Input: part model. Units: mm. Frame: model coordinates. A direction names the side the tool comes from. Give positions to 0.01 mm unless a question says otherwise; leave off trailing zeros. Loops run counter-clockwise (first coordinate to the right, second up) from the corner with the lowest first, then second, coordinate; pieces in that order, holes last. Notation, with made-up numbers: (35.5, 65.5) - (47.5, 65.5) arc R21 cw to (47.5, 91.5) - close; hole circle Ø3 at (39, 18.25). An arc over 180 degrees is marked (long way). Answer as a JSON object with one key per item and string values.
from build123d import *

# Parameters (mm, degrees)
SKETCH_2_R          = 2.5
CHAMFER_1_SIZE      = 10
CHAMFER_1_SIZE2     = 1.583844403
SKETCH_4_W          = 3.296860699
SKETCH_4_H          = 5.658889041
SKETCH_4_W_2        = 5.658889041
SKETCH_4_H_2        = 3.296860699
CUT_EXTRUDE_1_DEPTH = 40
DOME_1_FACE_RADIUS  = 0.916155597
DOME_1_HEIGHT       = 1


with BuildPart() as part:
    # 扫描1: sweep along a path in 草图1
    with BuildLine(Plane.XY) as sweep_1_path:
        Line((0, 0), (0, 34.641016151))
        ThreePointArc((0, 34.641016151), (0.681483474, 39.817397053), (2.679491924, 44.641016151))
        Line((2.679491924, 44.641016151), (17.5, 70.310889132))
    # 草图2 → 扫描1 (sweep)
    with BuildSketch(Plane(origin=(0, 0, 0), x_dir=(1, 0, 0), z_dir=(0, 1, 0))):
        Circle(SKETCH_2_R)
    sweep(path=sweep_1_path.line)

    # 草图3 → 旋转1 (revolve)
    with BuildSketch(Plane.XY, mode=Mode.PRIVATE) as revolve_1_sk:
        Polygon((0, 0), (2.5, 0), (4, -8), (4, -40), (0, -40), align=None)
    revolve(revolve_1_sk.sketch.rotate(Axis((0, 0, 0), (0, -1, 0)), 90), axis=Axis((0, 0, 0), (0, -1, 0)))

    # 倒角1
    chamfer_1_edges = [part.edges().sort_by_distance(p)[0] for p in [
        (15.334936491, 71.560889132, 0),
    ]]
    chamfer_1_side = [part.faces().sort_by_distance(p)[0] for p in [
        (7.924682453, 58.725952642, 0),
    ]]
    chamfer(chamfer_1_edges, length=CHAMFER_1_SIZE, length2=CHAMFER_1_SIZE2, reference=chamfer_1_side[0])

    # 草图4 → 切除-拉伸1 (cut)
    with BuildSketch(Plane.XZ.offset(40)):
        with Locations((5.148430349, -0.020531218)):
            Rectangle(SKETCH_4_W, SKETCH_4_H)
        with Locations((0.020531218, 5.148430349)):
            Rectangle(SKETCH_4_W_2, SKETCH_4_H_2)
        with Locations((-0.020531218, -5.148430349)):
            Rectangle(SKETCH_4_W_2, SKETCH_4_H_2)
        with Locations((-5.148430349, 0.020531218)):
            Rectangle(SKETCH_4_W, SKETCH_4_H)
    extrude(amount=-CUT_EXTRUDE_1_DEPTH, mode=Mode.SUBTRACT)

    # 圆顶1: a dome of height H over a round flat face of radius A is a cap of a sphere of radius (A * A + H * H) / (2 * H)
    dome_1_r = (DOME_1_FACE_RADIUS * DOME_1_FACE_RADIUS + DOME_1_HEIGHT * DOME_1_HEIGHT) / (2 * DOME_1_HEIGHT)
    dome_1_base = Plane((17.5, 70.310889132, 0), z_dir=(0.5, 0.866025403784, 0))
    with Locations(dome_1_base.offset(DOME_1_HEIGHT - dome_1_r)):
        dome_1_ball = Sphere(dome_1_r, mode=Mode.PRIVATE)
    add(split(dome_1_ball, bisect_by=dome_1_base, keep=Keep.TOP, mode=Mode.PRIVATE))


solid = part.part
Item 1: Material intervals for line 1 (X direction, y = -20.5, z = 0); line 2 (X direction, y = 12, z = 0); line 3 (Y direction, x = 11.5, z = -1), sorted ascending. Write a range as [from, to].
Geometry check:
{"line 1": "x = [-3.5, 3.5]", "line 2": "x = [-2.5, 2.5]", "line 3": "y = [55.34, 63.97]"}
Item 2: Cut plane B-B (z = 0). Return loops of the section in (x, y), then the cut area to 3 significant figures.
Geometry check:
{"outline": "(-3.5, -40) - (3.5, -40) - (3.5, -5.33) - (2.5, 0) - (2.5, 34.64) arc R17.5 cw to (4.84, 43.39) - (14.67, 60.4) - (18.29, 69.85) arc R0.92 ccw (long way) to (16.71, 70.77) - (10.33, 62.9) - (0.51, 45.89) arc R22.5 ccw to (-2.5, 34.64) - (-2.5, 0) - (-3.5, -5.33) - close", "area": "634 mm2"}
Item 3: Access query for faces 1 (the face through (16.393, 65.258, 0.65)), 2 (the face through (3.5, -23, 0)). Directions: +Z, -Z, +X, -X, +Y, -Y. A direction counts if a zero-diameter tool reaches every point of the face in a straight line with its end or side. Return the directions, or none.
Geometry check:
{"face 1": "none", "face 2": "+Z, -Z, +X, -Y"}
Item 4: Cut plane A-A (y = -29.5). Return loops of the section in (x, z), then the cut area to 3 significant figures.
Geometry check:
{"outline": "(-3.5, -1.94) arc R4 ccw to (-1.94, -3.5) - (1.94, -3.5) arc R4 ccw to (3.5, -1.94) - (3.5, 1.94) arc R4 ccw to (1.94, 3.5) - (-1.94, 3.5) arc R4 ccw to (-3.5, 1.94) - close", "area": "45.0 mm2"}
Item 5: Cut plane C-C (y = 11). Return loops of the section in (x, z), then the cut area to 3 significant figures.
Geometry check:
{"outline": "circle Ø5 at (0, 0)", "area": "19.6 mm2"}
Item 6: Contact query for flat-ended pins moving along their axis: P1, Ø2, axis at y = 59, z = 0.5, coming from the +X side; P2, Ø4, axis at x = 4.5, z = 1.5, coming from the +Y side; P3, Ø1.5, axis at x = 3.5, z = -0.5, coming from the +Y side. Output: stop coordinate, or through.
Geometry check:
{"P1": "stops at x = 14.4", "P2": "stops at y = 55.78", "P3": "stops at y = 52.29"}
Item 7: Mould query, pull axis Y, two halves, no side actions, for faces 3 (the face through (1.18, -3.17, 2.86)), 4 (the face through (-0.54, 17.56, 2.44)), 5 (the face through (0, -40, 0)), 6 (the face through (0, -23, -3.5)). Classes: released by +Y, released by -Y, zero draft, split by the parting line, or undercut.
Geometry check:
{"face 3": "undercut", "face 4": "undercut", "face 5": "released by -Y", "face 6": "zero draft"}
